Geometry: see drawing. Coordinates: mm, zero at the bounding-box minimum. Coordinates: 2 decimals unless noted, no trailing zeros. Write each loop counter-clockwise with the first axis right and the second up, starting at its lowest first coordinate (ties: lowest second). Pieces come first, ordered by that corner, then holes. Notation, with made-up numbers: (21, -4.75) - (69, -4.75) arc R14 cw to (69, 20.25) - close; hole circle Ø9 at (60.5, 4.5). An arc over 180 degrees is marked (long way). Use a Markdown table: item, result. Add a question column.
Q1. Section query C-C (y = 1.5). Return the cut outline in (x, z) (1 decimal), then the cut area to 3 significant figures.
Q2. Pin query (flat end, axial travel): P1, Ø1, axis at x = 13, z = 6.5, coming from the -Y side; P2, Ø1, axis at x = 19, y = 0.5, coming from the +Z side; P3, Ø1, axis at x = 23, y = 1, coming from the -Z side. Return the tip coordinate at first contact, or that it passes through.
Q3. Section query B-B (x = 3.25). Return the cut outline in (y, z).
Q4. Section query A-A (z = 12.75). Return the cut outline in (x, y) (1 decimal).
Q5. Mould query, pull axis X, two halves, no side actions, for the marked faces 1 and 2. Classes: released by +X, released by -X, zero draft, split by the parting line, or undercut.
Q6. Section query D-D (x = 18). Give the number of separate pieces and of enclosed holes in the cut face.
Q7. Material intervals for probe 1 along Z at (x, y) = (7, 1.45) (1 decimal); probe 2 along Z at (x, y) = (10, 1) (1 decimal); probe 3 along X at (y, z) = (1.85, 16) (1 decimal), sorted ascending. Write a range as from..to.
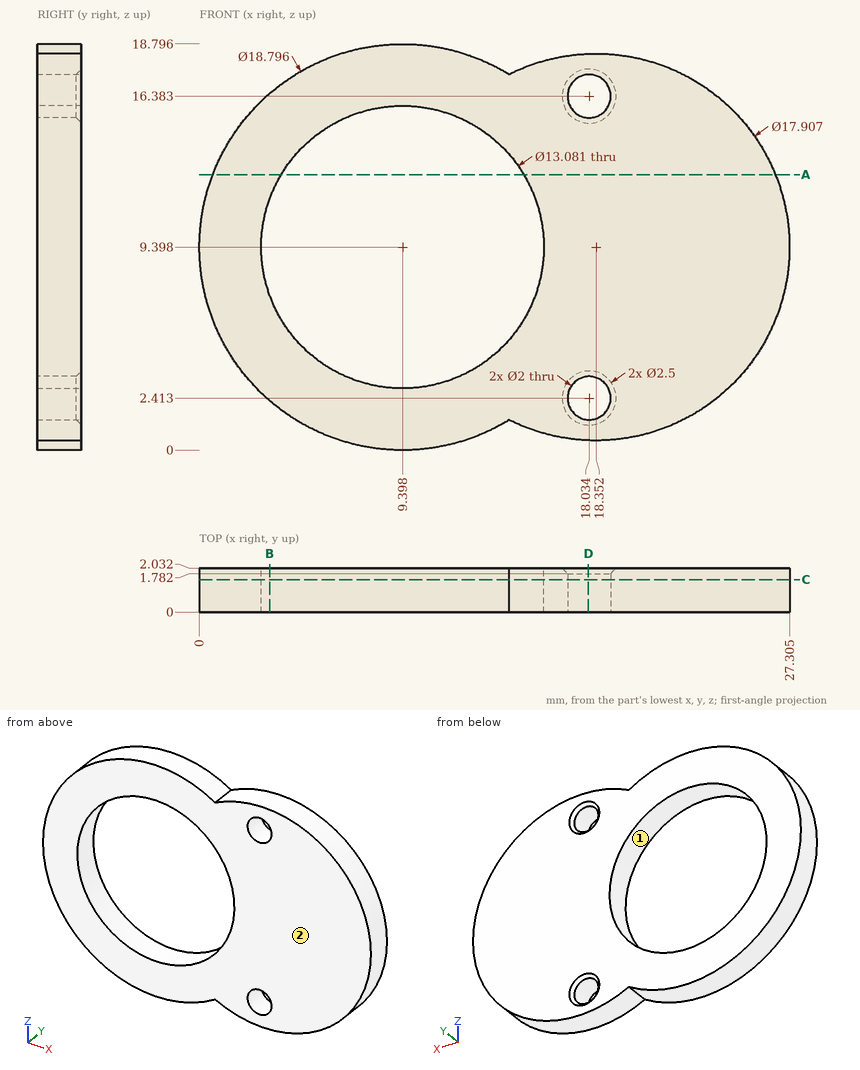
Values follow:
| question | item | result |
|---|---|---|
| 1 | outline | (14.3, 1.4) arc R9 ccw (long way) to (14.3, 17.4) arc R9.4 ccw (long way) to start; hole circle Ø13.1 at (9.4, 9.4); hole circle Ø2 at (18, 2.4); hole circle Ø2 at (18, 16.4) |
| 1 | area | 282 mm2 |
| 2 | P1 | through |
| 2 | P2 | z = 18.35 |
| 2 | P3 | z = 1.46 |
| 3 | outline | (0, 2.29) - (2.03, 2.29) - (2.03, 7.17) - (0, 7.17) - close; (0, 11.63) - (2.03, 11.63) - (2.03, 16.51) - (0, 16.51) - close |
| 4 | outline | (0.6, 0) - (3.8, 0) - (3.8, 2) - (0.6, 2) - close; (15, 0) - (26.7, 0) - (26.7, 2) - (15, 2) - close |
| 5 | face 1 | undercut |
| 5 | face 2 | zero draft |
| 6 | separate pieces | 3 |
| 6 | enclosed holes | 0 |
| 7 | probe 1 | 0.3..3.3, 15.5..18.5 |
| 7 | probe 2 | 0..2.9, 15.9..18.8 |
| 7 | probe 3 | 2.7..17, 19..24.4 |
